```python
from build123d import *

# Parameters (mm, degrees)
SKETCH2_R           = 15.875
BOSS_EXTRUDE1_DEPTH = 6.35
FILLET1_R           = 6.35


with BuildPart() as part:
    # Sketch2 → Boss-Extrude1 (new body)
    with BuildSketch(Plane.XY):
        Polygon((0, 0), (-165.1, 0), (-165.1, 34.925), (-285.75, 34.925), (-285.75, -57.15), (-412.75, -57.15), (-412.75, 393.7), (0, 393.7), align=None)
        with Locations((-63.5, 63.5)):
            Circle(SKETCH2_R, mode=Mode.SUBTRACT)
    extrude(amount=BOSS_EXTRUDE1_DEPTH)

    # Fillet1
    fillet1_edges = [part.edges().sort_by_distance(p)[0] for p in [
        (-412.75, 393.7, 3.175),
        (0, 393.7, 3.175),
        (0, 0, 3.175),
        (-165.1, 0, 3.175),
        (-165.1, 34.925, 3.175),
        (-285.75, 34.925, 3.175),
        (-285.75, -57.15, 3.175),
    ]]
    fillet(fillet1_edges, radius=FILLET1_R)


solid = part.part
```
Design review of the part built by this model. Coordinates are the model's own, in mm. Give positions to 0.01 mm unless a question says otherwise; leave off trailing zeros. Order: outer loops, then holes, each group sorted by start corner. A loop starts at its lowest first (then second) coordinate and runs counter-clockwise, first axis right, second up. Notation, with made-up numbers: (0.5, -32.75) - (16.5, -32.75) arc R7 cw to (16.5, -25.75) - close; hole circle Ø8 at (66.5, 16.25). An arc over 180 degrees is marked (long way). Use a Markdown table: item, result. Add a question column.
(1) Mouldability with a two-part tool opening along Y and no side actions: class faces 1 (the face through (-48.836, 57.42, 3.131)), 2 (the face through (-203, 171, 6.35)) as +Y half, -Y half, draft (parallel to the pull), parting line (faces both ways), or undercut.
(2) Add section B-B on y = 63.5. Give the boundary of the cut face in (x, z) (3 decimals).
(3) Add section D-D on x = -250. Give the boundary of the cut face in (y, z) (3 decimals).
(4) Add section A-A on x = -63.5. Give the boundary of the cut face in (y, z) (3 decimals), then the cut area to 3 significant figures.
(5) Clearance check with flat-ended pins moving along their axes: P1, Ø1.9, axis at y = -6, z = 3, coming from the +X side; P2, Ø2, axis at x = -325, y = 307.5, coming from the -Z side; P3, Ø3, axis at x = -236.5, z = 3.5, coming from the -Y side (3 decimals). State where each tip first meets the part, or that it passes through.
(6) Wall thickness on probe 1 along Y at (x, z) = (-63.5, 1.5) (3 decimals); probe 2 along Y at (x, z) = (-224, 2.5) (3 decimals); probe 3 along X at (y, z) = (-22, 3.75): over which ranges is each line inside the solid? List them lowest first. Write a range as [from, to].
(7) Add section C-C on z = 4.5. Give the boundary of the cut face in (x, y) (3 decimals).
Report:
| question | item | result |
|---|---|---|
| 1 | face 1 | undercut |
| 1 | face 2 | draft |
| 2 | outline | (-412.75, 0) - (-79.375, 0) - (-79.375, 6.35) - (-412.75, 6.35) - close; (-47.625, 0) - (0, 0) - (0, 6.35) - (-47.625, 6.35) - close |
| 3 | outline | (34.925, 0) - (393.7, 0) - (393.7, 6.35) - (34.925, 6.35) - close |
| 4 | outline | (0, 0) - (47.625, 0) - (47.625, 6.35) - (0, 6.35) - close; (79.375, 0) - (393.7, 0) - (393.7, 6.35) - (79.375, 6.35) - close |
| 4 | area | 2,300 mm² |
| 5 | P1 | stops at x = -285.75 |
| 5 | P2 | stops at z = 0 |
| 5 | P3 | stops at y = 34.925 |
| 6 | probe 1 | y = [0, 47.625], [79.375, 393.7] |
| 6 | probe 2 | y = [34.925, 393.7] |
| 6 | probe 3 | x = [-412.75, -285.75] |
| 7 | outline | (-412.75, -57.15) - (-292.1, -57.15) arc R6.35 ccw to (-285.75, -50.8) - (-285.75, 28.575) arc R6.35 cw to (-279.4, 34.925) - (-171.45, 34.925) arc R6.35 cw to (-165.1, 28.575) - (-165.1, 6.35) arc R6.35 ccw to (-158.75, 0) - (-6.35, 0) arc R6.35 ccw to (0, 6.35) - (0, 387.35) arc R6.35 ccw to (-6.35, 393.7) - (-406.4, 393.7) arc R6.35 ccw to (-412.75, 387.35) - close; hole circle Ø31.75 at (-63.5, 63.5) |
